```python
from build123d import *

# Parameters (mm, degrees)
F0_W     = 30
F0_H     = 40
F0_R     = 3
F1_DEPTH = 4
F3_DEPTH = 20
F5_DEPTH = 30.001
F6_SIZE  = 5
F8_DEPTH = 33.321
F9_SIZE2 = 2
F9_SIZE  = 2
F10_SIZE = 1


with BuildPart() as f1:
    # F0 (on Top) → F1 (new body)
    with BuildSketch(Plane.XY):
        Rectangle(F0_W, F0_H)
        Circle(F0_R, mode=Mode.SUBTRACT)
    extrude(amount=F1_DEPTH)

    # F2 (on face) → F3 (join)
    with BuildSketch(Plane.XY.offset(4)):
        Polygon((-15, 9.32), (15, 9.32), (15, 13.32), (10, 13.32), (10, 20), (6, 20), (6, 13.32), (-6, 13.32), (-6, 20), (-10, 20), (-10, 13.32), (-15, 13.32), align=None)
        Polygon((15, -13.32), (15, -9.32), (-15, -9.32), (-15, -13.32), (-10, -13.32), (-10, -20), (-6, -20), (-6, -13.32), (6, -13.32), (6, -20), (10, -20), (10, -13.32), align=None)
    extrude(amount=F3_DEPTH)

    # F4 (on face) → F5 (cut, through all)
    with BuildSketch(Plane(origin=(-15, 0, 0), x_dir=(0, -1, 0), z_dir=(-1, 0, 0))):
        Polygon((-20, 24), (-20, 4), (-13.32, 24), align=None)
        Polygon((20, 24), (13.32, 24), (20, 4), align=None)
    extrude(amount=-F5_DEPTH, mode=Mode.SUBTRACT)

    # F6
    f6_edges = [f1.edges().sort_by_distance(p)[0] for p in [
        (-15, 20, 2),
        (-15, -20, 2),
        (15, 20, 2),
        (15, -20, 2),
        (-15, 11.32, 24),
        (-15, -11.32, 24),
        (15, -11.32, 24),
        (15, 11.32, 24),
    ]]
    chamfer(f6_edges, length=F6_SIZE)

    # F7 (on face) → F8 (cut, through all)
    with BuildSketch(Plane.XZ.offset(13.32)):
        Polygon((0, 14), (-3, 4), (3, 4), align=None)
    extrude(amount=-F8_DEPTH, mode=Mode.SUBTRACT)

    # F9
    f9_edges = [f1.edges().sort_by_distance(p)[0] for p in [
        (-1.5, -13.32, 9),
        (1.5, -13.32, 9),
        (1.5, 13.32, 9),
        (-1.5, 13.32, 9),
    ]]
    chamfer(f9_edges, length=F9_SIZE, length2=F9_SIZE2)

    # F10
    f10_edges = [f1.edges().sort_by_distance(p)[0] for p in [
        (15, -9.32, 11.5),
        (12.5, -9.32, 21.5),
        (0, -9.32, 24),
        (-15, -9.32, 11.5),
        (-12.5, -9.32, 21.5),
        (-15, 9.32, 11.5),
        (-12.5, 9.32, 21.5),
        (0, 9.32, 24),
        (12.5, 9.32, 21.5),
        (15, 9.32, 11.5),
    ]]
    chamfer(f10_edges, length=F10_SIZE)


solid = f1.part
```
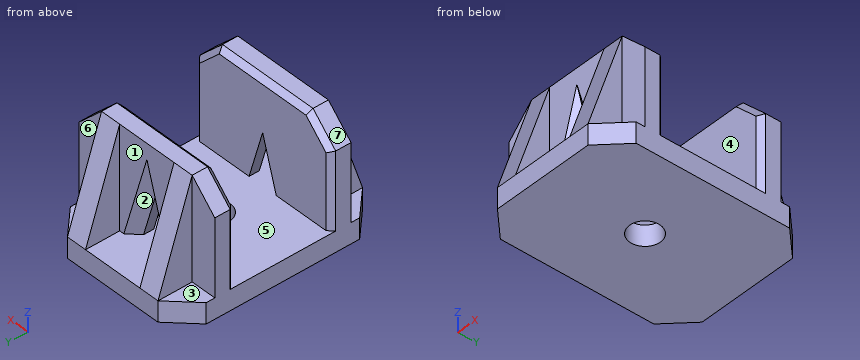
The model under review builds one solid part; all positions refer to its coordinate system, in mm. Face numbers are marked on the shaded views. A direction names the side the tool comes from. Round coordinates to 2 decimals unless told otherwise and drop trailing zeros. Loops run counter-clockwise (first coordinate to the right, second up) from the corner with the lowest first, then second, coordinate; pieces in that order, holes last. Notation, with made-up numbers: M 55.25,-11.5 L 105.25,-11.5 A24 ccw 105.25,10.5 Z; hole C 18,88.25 d6. An arc over 180 degrees is marked long. Put each result on its own line as item: value.
Q1. Mouldability with a two-part tool opening along X and no side actions: class the marked faces 5, 6 and 7 as released by +X, released by -X, zero draft, split by the parting line, or undercut.
Result set:
face 5: undercut
face 6: zero draft
face 7: released by -X
Q2. Consider section C-C, the plane x = -6.5. Give the boundary of the cut face in (y, z).
Result set:
outline: M -20,0 L 20,0 L 20,4 L 13.32,24 L 10.32,24 L 9.32,23 L 9.32,4 L -9.32,4 L -9.32,23 L -10.32,24 L -13.32,24 L -20,4 Z
Q3. Consider section B-B, the plane x = 0.5. Give the boundary of the cut face in (y, z), then the cut area to 3 significant figures.
Result set:
outline: M -20,0 L -2.96,0 L -2.96,4 L -20,4 Z; M -13.32,19.29 L -11.32,12.33 L -9.32,12.33 L -9.32,23 L -10.32,24 L -13.32,24 Z; M 2.96,0 L 20,0 L 20,4 L 2.96,4 Z; M 9.32,12.33 L 11.32,12.33 L 13.32,19.29 L 13.32,24 L 10.32,24 L 9.32,23 Z
area: 215 mm²
Q4. Machinability: for the marked faces 1, 2, 3 and 4, which of the approach directions +Z, -Z, +X, -X, +Y, -Y give a long, thin tool a straight path to every point of the face, cutting with its end or side? Answer none if there is none.
Result set:
face 1: +Z, +Y
face 2: +Y
face 3: +Z, -X, +Y
face 4: +Z, +X, -X
Q5. To check wall thickness, follow L1, parallel to Y at x = 13, z = 11; L2, parallel to Y at x = 0, z = 2.75; L3, parallel to X at y = 0, z = 2.2. State the ranges of each line that lie inside material, in increasing order.
Result set:
L1: y = -13.32 to -9.32, 9.32 to 13.32
L2: y = -20 to -3, 3 to 20
L3: x = -15 to -3, 3 to 15
Q6. Consider section D-D, the plane y = -16.5. Give the boundary of the cut face in (x, z).
Result set:
outline: M -13.5,0 L 13.5,0 L 13.5,4 L 10,4 L 10,14.48 L 6,14.48 L 6,4 L -6,4 L -6,14.48 L -10,14.48 L -10,4 L -13.5,4 Z
Q7. Consider section A-A, the plane y = 0. Give the boundary of the cut face in (x, z).
Result set:
outline: M -15,0 L -3,0 L -3,4 L -15,4 Z; M 3,0 L 15,0 L 15,4 L 3,4 Z
Q8. For pin 1 (10 mm diameter, centred on y = -2, z = 18.5, fed in from -X); pin 2 (6 mm diameter, centred on x = -3, y = -4, fed in from -Z); pin 3 (2.5 mm diameter, centred on x = 12, z = 11.5, fed in from -Y); pin 4 (6 mm diameter, centred on x = -6, z = 19.5, fed in from -Y) (3 decimals), all flat-tipped, find the tip position at first contact; note any pin that passes through.
Result set:
pin 1: passes through
pin 2: stops at z = 0
pin 3: stops at y = -13.32
pin 4: stops at y = -15.825
